```python
from build123d import *

# Parameters (mm, degrees)
F0_W     = 148.923736
F0_H     = 105.609175
F1_DEPTH = 29.464
F2_R     = 24.768688
F3_DEPTH = 51.308
F5_DEPTH = 1143


with BuildPart() as f1:
    # F0 (on Top) → F1 (new body)
    with BuildSketch(Plane.XY):
        with Locations((16.5732, 5.461818)):
            Rectangle(F0_W, F0_H)
    extrude(amount=F1_DEPTH)

    # F2 (on face) → F3 (join)
    with BuildSketch(Plane.XY.offset(29.464)):
        with Locations((15.579882, 5.789573)):
            Circle(F2_R)
    extrude(amount=F3_DEPTH)

    # F4 (on Front) → F5 (cut, symmetric)
    with BuildSketch(Plane.XZ):
        Polygon((40.655378, 84.109753), (-16.463115, 84.109753), (40.655378, 46.179499), align=None)
    extrude(amount=F5_DEPTH, both=True, mode=Mode.SUBTRACT)


solid = f1.part
```
Can you work these out from the model? Positions are in its coordinate system, mm. A direction names the side the tool comes from. Coordinates: 2 decimals unless noted, no trailing zeros. Write each loop counter-clockwise with the first axis right and the second up, starting at its lowest first coordinate (ties: lowest second). Pieces come first, ordered by that corner, then holes. Notation, with made-up numbers: M 55,33.25 L 62,33.25 A11 ccw 62,38.25 Z; hole C -16.75,18 d11. An arc over 180 degrees is marked long. Write item = value, one per line. Start each with the question number.
Q1. If I drill on L1, parallel to Y at x = 14.5, z = 62.5; L2, parallel to Z at x = 60, y = -9; L3, parallel to X at y = 10, z = 62.5, over which ranges is the centre line in solid material (lowest first)? Write a range as [from, to].
Q2. On a 3-axis mill with a long thin cutter (end or side, diameter ignored), from which of +Z, -Z, +X, -X, +Y, -Y can I reach the whole of each face in a straight line? I mean faces 4 (the face through (-9.165, 6.879, 48.748)), 5 (the face through (16, 58.266, 15)). Say none if no direction works.
Q3. If we section it at C-C, the plane z = 58: Write out the boundary of the cut face in (x, y).
Q4. I'm going to push flat-ended pins straight in: pin 1 (5 mm diameter, centred on x = 17.5, y = 35.5, fed in from +Z); pin 2 (12 mm diameter, centred on x = 0, z = 60, fed in from -Y). Where does each tip first touch, or does it pass through?
Q5. Thinking about a two-plate mould opening in Z: for faces 1 (the face through (91.035, 5, 15)), 2 (the face through (-1, 30, 29.464)), 3 (the face through (16, 6, 0)), which applies, released by +Z, released by -Z, zero draft, split by the parting line, or undercut?
Q6. If we section it at D-D, the plane y = 42: Write out the boundary of the cut face in (x, z), then the cut area to 3 significant figures.
Q7. If we section it at A-A, the plane y = 22.5: Write out the boundary of the cut face in (x, z).
Q8. If we section it at B-B, the plane x = 24.5: Write out the boundary of the cut face in (y, z).
Check sheet entries:
q1.L1 = [-18.96, 30.53]
q1.L2 = [0, 29.46]
q1.L3 = [-8.83, 16.08]
q2.face_4 = +Z
q2.face_5 = +Z, -Z, +X, -X, +Y
q3.outline = M 22.86,-17.89 L 22.86,29.47 A24.77 ccw long Z
q4.pin_1 = 29.46
q4.pin_2 = -17.05
q5.face_1 = zero draft
q5.face_2 = released by +Z
q5.face_3 = released by -Z
q6.outline = M -57.89,0 L 91.04,0 L 91.04,29.46 L -57.89,29.46 Z
q6.area = 4,390 mm²
q7.outline = M -57.89,0 L 91.04,0 L 91.04,29.46 L 33.86,29.46 L 33.86,50.69 L -2.7,74.97 L -2.7,29.46 L -57.89,29.46 Z
q8.outline = M -47.34,0 L 58.27,0 L 58.27,29.46 L 28.9,29.46 L 28.9,56.91 L -17.32,56.91 L -17.32,29.46 L -47.34,29.46 Z
